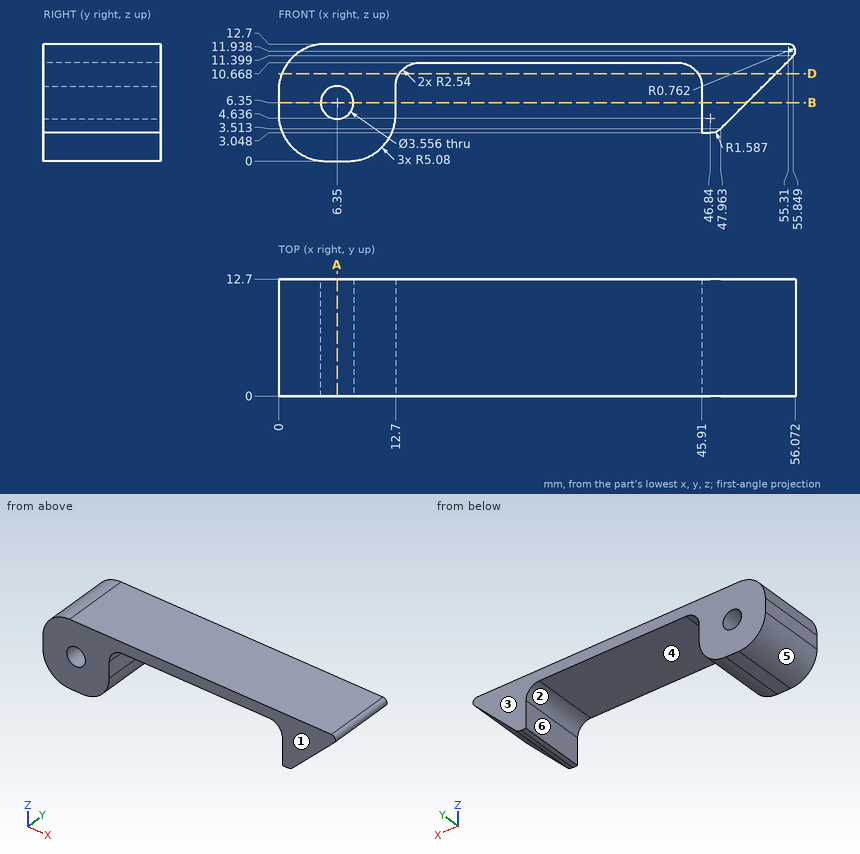
Can you work these out from the drawing? Everything is in mm from the part's minimum corner. A direction names the side the tool comes from. Coordinates: 2 decimals unless noted, no trailing zeros. Loops run counter-clockwise (first coordinate to the right, second up) from the corner with the lowest first, then second, coordinate; pieces in that order, holes last. Notation, with made-up numbers: (26, 68.5) - (38, 68.5) arc R32 ccw to (38, 102.5) - close; hole circle Ø5 at (-4, 27.5). An arc over 180 degrees is marked (long way). Put each result on its own line as item: value. Start each with the question number.
Item 1: Which directions (+Z, -Z, +X, -X, +Y, -Y) give clear straight access to the entire face, cutting with the end or side of a thin tool? Please do the marked faces 1 and 2.
Item 2: Suppose I cut it at D-D (z = 9.5). Please give me the cut outline in (x, y), and give its area (3 significant figures).
Item 3: Suppose I cut it at B-B (z = 6.35). Please give me the cut outline in (x, y), and give its area (3 significant figures).
Item 4: For pin 1 (0.5 mm diameter, centred on x = 46.5, y = 8.5, fed in from -Z); pin 2 (4 mm diameter, centred on x = 32.5, y = 7, fed in from -Z); pin 3 (3.5 mm diameter, centred on y = 8, z = 7.5, fed in from +X); pin 4 (2 mm diameter, centred on x = 6.35, z = 6.35, fed in from -Y), each with a flat end and sliding along its axis, tell me the tip position at first contact or that it passes through.
Item 5: Suppose I cut it at A-A (x = 6.35). Please give me the cut outline in (y, z), and give its area (3 significant figures).
Item 6: If we mould it in two halves opening along X, with no side actions, what happens to the marked faces 3, 4, 5 and 6? For each: +X half, -X half, draft (parallel to the pull), parting line (faces both ways), or undercut.
Item 7: If I drill on line 1 along Z through (x, y) = (6.35, 7.5); line 2 along X through (y, z) = (10, 4.75) (1 decimal); line 3 along Z through (x, y) = (28, 9.75), over which ranges is the centre line in solid material (lowest first)?
Here are the results:
1. face 1: +Z, -Z, +X, -X, -Y
1. face 2: -Z, +Y, -Y
2. outline: (0.36, 0) - (13.1, 0) - (13.1, 12.7) - (0.36, 12.7) - close; (45.51, 0) - (53.95, 0) - (53.95, 12.7) - (45.51, 12.7) - close
2. area: 269 mm²
3. outline: (0, 0) - (4.57, 0) - (4.57, 12.7) - (0, 12.7) - close; (8.13, 0) - (12.7, 0) - (12.7, 12.7) - (8.13, 12.7) - close; (45.91, 0) - (50.8, 0) - (50.8, 12.7) - (45.91, 12.7) - close
3. area: 178 mm²
4. pin 1: z = 3.05
4. pin 2: z = 10.67
4. pin 3: x = 53.7
4. pin 4: through
5. outline: (0, 0) - (12.7, 0) - (12.7, 4.57) - (0, 4.57) - close; (0, 8.13) - (12.7, 8.13) - (12.7, 12.7) - (0, 12.7) - close
5. area: 116 mm²
6. face 3: draft
6. face 4: undercut
6. face 5: -X half
6. face 6: undercut
7. line 1: 0 to 4.57, 8.13 to 12.7
7. line 2: 0 to 5.6, 7.1 to 12.7, 45.9 to 49.2
7. line 3: 10.67 to 12.7
